The model under review builds one solid part; all positions refer to its coordinate system, in mm. Face numbers are marked on the shaded views. A direction names the side the tool comes from. Round coordinates to 2 decimals unless told otherwise and drop trailing zeros. Write each loop counter-clockwise with the first axis right and the second up, starting at its lowest first coordinate (ties: lowest second). Pieces come first, ordered by that corner, then holes. Notation, with made-up numbers: M 9,47 L 25,47 A25 cw 25,63 Z; hole C 49.25,39.25 d10. An arc over 180 degrees is marked long. One line per item, written item: value. Start each with the question number.
1) Wall thickness on probe 1 along Z at (x, y) = (13, 4.8); probe 2 along X at (y, z) = (2.8, 9); probe 3 along Z at (x, y) = (7, 1.75): over which ranges is each line inside the solid? List them lowest first.
2) For P1, Ø0.8, axis at y = 1, z = -14, coming from the +X side; P2, Ø1, axis at y = 4, z = -7.5, coming from the +X side; P3, Ø1.2, axis at x = -13.5, z = -8, coming from the +Y side, all flat-tipped, find the tip position at first contact; note any pin that passes through.
3) Take a section at A-A, the plane x = -2.5. Write out the cut boundary in (y, z), and give its area (3 significant figures).
4) Mouldability with a two-part tool opening along X and no side actions: class the marked faces 1, 2 and 3 as +X half, -X half, draft (parallel to the pull), parting line (faces both ways), or undercut.
5) Take a section at C-C, the plane z = -9.5. State how many separate pieces and enclosed holes the cut face has, and give its area (3 significant figures).
6) Tool access review of the marked faces 4, 5 and 6: name each direction out of +Z, -Z, +X, -X, +Y, -Y from which nothing blocks a thin tool from reaching the whole face with its end or side.
7) Take a section at B-B, the plane z = 4.5. Write out the cut boundary in (x, y).
8) Take a section at D-D, the plane z = -0.5. Write out the cut boundary in (x, y), and give its area (3 significant figures).
from build123d import *

# Parameters (mm, degrees)
SKETCH1_W           = 32
SKETCH1_H           = 29
BOSS_EXTRUDE1_DEPTH = 6
SKETCH2_R           = 1
CUT_EXTRUDE1_DEPTH  = 10
SKETCH3_W           = 21
SKETCH3_H           = 9.6
CUT_EXTRUDE2_DEPTH  = 10
SKETCH4_W           = 31
SKETCH4_H           = 27
CUT_EXTRUDE3_DEPTH  = 1
FILLET2_R           = 3
SKETCH5_R           = 2
CUT_EXTRUDE4_DEPTH  = 2
CHAMFER2_SIZE       = 1
SKETCH6_W           = 1
SKETCH6_H           = 11
CUT_EXTRUDE5_DEPTH  = 2.5
FILLET3_R           = 0.3
SKETCH7_W           = 31
SKETCH7_H           = 13
CUT_EXTRUDE6_DEPTH  = 2.5
FILLET4_R           = 1
SKETCH_1_W          = 21
SKETCH_1_H          = 12.05
CUT_EXTRUDE_1_DEPTH = 2.5
FILLET_1_R          = 1
SKETCH_2_W          = 11
SKETCH_2_H          = 2.5
CUT_EXTRUDE_2_DEPTH = 33.802439001
FILLET_2_R          = 0.3


with BuildPart() as part:
    # Sketch1 → Boss-Extrude1 (new body)
    with BuildSketch(Plane(origin=(0, 0, 0), x_dir=(1, 0, 0), z_dir=(0, 1, 0))):
        Rectangle(SKETCH1_W, SKETCH1_H)
    extrude(amount=BOSS_EXTRUDE1_DEPTH)

    # Sketch2 → Cut-Extrude1 (cut)
    with BuildSketch(Plane(origin=(0, 6, 0), x_dir=(1, 0, 0), z_dir=(0, 1, 0))):
        with Locations(Location((-13, 9, 0), (0, 0, 270))):
            Circle(SKETCH2_R)
        with Locations(Location((13, 9, 0), (0, 0, 270))):
            Circle(SKETCH2_R)
        with Locations(Location((13, -9, 0), (0, 0, 270))):
            Circle(SKETCH2_R)
        with Locations(Location((-13, -9, 0), (0, 0, 270))):
            Circle(SKETCH2_R)
    extrude(amount=-CUT_EXTRUDE1_DEPTH, mode=Mode.SUBTRACT)

    # Sketch3 → Cut-Extrude2 (cut)
    with BuildSketch(Plane(origin=(0, 6, 0), x_dir=(1, 0, 0), z_dir=(0, 1, 0))):
        with Locations((0, -6.25)):
            Rectangle(SKETCH3_W, SKETCH3_H)
    extrude(amount=-CUT_EXTRUDE2_DEPTH, mode=Mode.SUBTRACT)

    # Sketch4 → Cut-Extrude3 (cut)
    with BuildSketch(Plane.XZ):
        Rectangle(SKETCH4_W, SKETCH4_H)
    extrude(amount=-CUT_EXTRUDE3_DEPTH, mode=Mode.SUBTRACT)

    # Fillet2
    # the kernel refuses this fillet: 3 mm, written as the material it takes off along each edge
    with BuildSketch(Plane(origin=(16, 6, 22), x_dir=(0, -1, 0), z_dir=(0, 0, -1)), Plane(origin=(-16, 6, -22), x_dir=(0, -1, 0), z_dir=(0, 0, 1))) as fillet2_piece_1:
        with BuildLine():
            CenterArc((FILLET2_R, FILLET2_R), FILLET2_R, 180, 90)
            Line((0, FILLET2_R), (0, 0))
            Line((0, 0), (FILLET2_R, 0))
        make_face()
    extrude(amount=44, mode=Mode.SUBTRACT)

    # Sketch5 → Cut-Extrude4 (cut)
    with BuildSketch(Plane(origin=(0, 6, 0), x_dir=(1, 0, 0), z_dir=(0, 1, 0))):
        with Locations(Location((-13, 9, 0), (0, 0, 270))):
            Circle(SKETCH5_R)
        with Locations(Location((13, 9, 0), (0, 0, 270))):
            Circle(SKETCH5_R)
        with Locations(Location((13, -9, 0), (0, 0, 270))):
            Circle(SKETCH5_R)
        with Locations(Location((-13, -9, 0), (0, 0, 270))):
            Circle(SKETCH5_R)
    extrude(amount=-CUT_EXTRUDE4_DEPTH, mode=Mode.SUBTRACT)

    # Chamfer2
    chamfer2_edges = [part.edges().sort_by_distance(p)[0] for p in [
        (16, 1.5, 14.5),
        (15.121320344, 5.121320344, 14.5),
        (-15.121320344, 5.121320344, 14.5),
        (-16, 1.5, 14.5),
        (-16, 1.5, -14.5),
        (0, 6, -14.5),
        (16, 1.5, -14.5),
        (15.121320344, 5.121320344, -14.5),
        (-15.121320344, 5.121320344, -14.5),
        (0, 6, 14.5),
    ]]
    chamfer(chamfer2_edges, length=CHAMFER2_SIZE)

    # Sketch6 → Cut-Extrude5 (cut)
    with BuildSketch(Plane.XZ):
        with Locations((-15.5, 0)):
            Rectangle(SKETCH6_W, SKETCH6_H)
        with Locations((15.5, 0)):
            Rectangle(SKETCH6_W, SKETCH6_H)
    extrude(amount=-CUT_EXTRUDE5_DEPTH, mode=Mode.SUBTRACT)

    # Fillet3
    fillet3_edges = [part.edges().sort_by_distance(p)[0] for p in [
        (-15.5, 2.5, 5.5),
        (-15.5, 2.5, -5.5),
        (15.5, 2.5, -5.5),
        (15.5, 2.5, 5.5),
    ]]
    fillet(fillet3_edges, radius=FILLET3_R)

    # Sketch7 → Cut-Extrude6 (cut)
    with BuildSketch(Plane.XZ.offset(-1)):
        Rectangle(SKETCH7_W, SKETCH7_H)
    extrude(amount=-CUT_EXTRUDE6_DEPTH, mode=Mode.SUBTRACT)

    # Fillet4
    fillet4_edges = [part.edges().sort_by_distance(p)[0] for p in [
        (-13, 3.5, 6.5),
        (13, 3.5, 6.5),
        (0, 3.5, -6.5),
    ]]
    fillet(fillet4_edges, radius=FILLET4_R)

    # Эскиз1 → Вырез-Вытянуть1 (cut)
    with BuildSketch(Plane.XZ.offset(-1)):
        with Locations((0, -7.475)):
            Rectangle(SKETCH_1_W, SKETCH_1_H)
    extrude(amount=-CUT_EXTRUDE_1_DEPTH, mode=Mode.SUBTRACT)

    # Скругление1
    fillet_1_edges = [part.edges().sort_by_distance(p)[0] for p in [
        (10.5, 3.5, -9.5),
        (-10.5, 3.5, -9.5),
    ]]
    fillet(fillet_1_edges, radius=FILLET_1_R)

    # Эскиз2 → Вырез-Вытянуть2 (cut, through all)
    with BuildSketch(Plane.XY.offset(-13.5)):
        with Locations((0, 1.25)):
            Rectangle(SKETCH_2_W, SKETCH_2_H)
    extrude(amount=-CUT_EXTRUDE_2_DEPTH, mode=Mode.SUBTRACT)

    # Скругление2
    fillet_2_edges = [part.edges().sort_by_distance(p)[0] for p in [
        (5.5, 2.5, -14),
        (-5.5, 2.5, -14),
    ]]
    fillet(fillet_2_edges, radius=FILLET_2_R)


solid = part.part
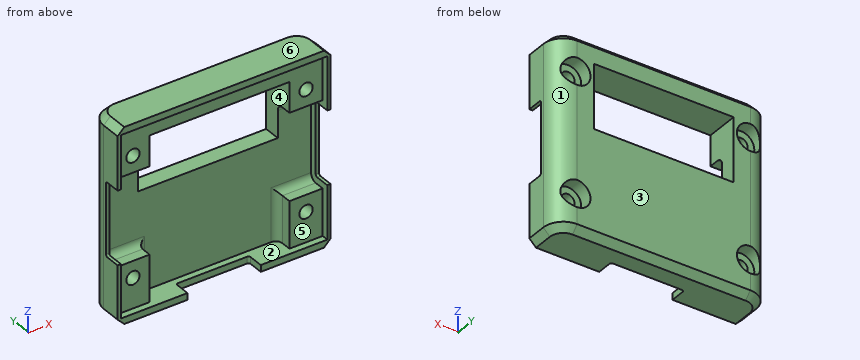
Checked values:
1. probe 1: z = -14.5 to -11, -7 to 7, 11 to 14.5
1. probe 2: x = -16 to -14, -12 to -10.5, 10.5 to 12, 14 to 16
1. probe 3: z = -14.5 to -13.5, 11.05 to 14.5
2. P1: stops at x = 15.9
2. P2: stops at x = 15.96
2. P3: stops at y = 4
3. outline: M 0,13.5 L 1,13.5 L 1,11.05 L 6,11.05 L 6,13.5 L 5,14.5 L 0,14.5 Z; M 2.5,-14.5 L 5,-14.5 L 6,-13.5 L 6,1.45 L 3.5,1.45 L 3.5,-13.5 L 2.5,-13.5 Z
3. area: 58.1 mm2
4. face 1: +X half
4. face 2: undercut
4. face 3: draft
5. separate pieces: 3
5. enclosed holes: 0
5. area: 80.0 mm2
6. face 4: +Y, -Y
6. face 5: -Y
6. face 6: +Z, +X, -X, +Y, -Y
7. outline: M -16,2.5 L -15.5,2.5 L -15.5,3.5 L -10.5,3.5 L -10.5,6 L -13,6 A3 ccw -16,3 Z; M 10.5,3.5 L 15.5,3.5 L 15.5,2.5 L 16,2.5 L 16,3 A3 ccw 13,6 L 10.5,6 Z
8. outline: M -16,2.5 L -15.5,2.5 L -15.5,3.5 L 15.5,3.5 L 15.5,2.5 L 16,2.5 L 16,3 A3 ccw 13,6 L -13,6 A3 ccw -16,3 Z
8. area: 77.1 mm2
